```python
from build123d import *

# Parameters (mm, degrees)
SKETCH1_W           = 109.4
SKETCH1_H           = 109.4
SKETCH1_W_2         = 79.4
SKETCH1_H_2         = 79.4
SKETCH1_R           = 6
SKETCH1_R_2         = 1.5
BOSS_EXTRUDE1_DEPTH = 8
BOSS_EXTRUDE2_DEPTH = 109.4
FILLET1_R           = 30
SKETCH5_W           = 8
SKETCH5_H           = 149.4
BOSS_EXTRUDE3_DEPTH = 109.4
SKETCH3_W           = 8
SKETCH3_H           = 109.4
CUT_EXTRUDE4_DEPTH  = 135
SKETCH7_W           = 8
SKETCH7_H           = 40
CUT_EXTRUDE5_DEPTH  = 135
SKETCH4_R           = 2.5
CUT_EXTRUDE6_DEPTH  = 10


with BuildPart() as part:
    # Sketch1 → Boss-Extrude1 (new body)
    # profile 1 of 2: a face of its own
    with BuildSketch(Plane.XY):
        with Locations((-17.5, 17.5)):
            Rectangle(SKETCH1_W, SKETCH1_H)
        with Locations((-17.5, 17.5)):
            Rectangle(SKETCH1_W_2, SKETCH1_H_2, mode=Mode.SUBTRACT)
    # profile 2 of 2: a face of its own
    with BuildSketch(Plane.XY):
        with Locations((-17.5, 17.5)):
            Rectangle(SKETCH1_W_2, SKETCH1_H_2)
        with Locations((-35, 0)):
            Circle(SKETCH1_R, mode=Mode.SUBTRACT)
        Circle(SKETCH1_R, mode=Mode.SUBTRACT)
        with Locations((0, 35)):
            Circle(SKETCH1_R, mode=Mode.SUBTRACT)
        with Locations((-35, 35)):
            Circle(SKETCH1_R, mode=Mode.SUBTRACT)
        with Locations((-52.809903828, -17.809903828)):
            Circle(SKETCH1_R_2, mode=Mode.SUBTRACT)
        with Locations((-17.5, -17.5)):
            Circle(SKETCH1_R_2, mode=Mode.SUBTRACT)
        with Locations((17.5, -17.5)):
            Circle(SKETCH1_R_2, mode=Mode.SUBTRACT)
        with Locations((17.5, 17.5)):
            Circle(SKETCH1_R_2, mode=Mode.SUBTRACT)
        with Locations((-17.5, 17.5)):
            Circle(SKETCH1_R_2, mode=Mode.SUBTRACT)
        with Locations((-52.5, 17.5)):
            Circle(SKETCH1_R_2, mode=Mode.SUBTRACT)
        with Locations((17.5, 52.5)):
            Circle(SKETCH1_R_2, mode=Mode.SUBTRACT)
        with Locations((-17.5, 52.5)):
            Circle(SKETCH1_R_2, mode=Mode.SUBTRACT)
        with Locations((-52.5, 52.5)):
            Circle(SKETCH1_R_2, mode=Mode.SUBTRACT)
    extrude(amount=BOSS_EXTRUDE1_DEPTH)



with BuildPart() as body_2:
    # Sketch2 → Boss-Extrude2 (new body)
    with BuildSketch(Plane(origin=(37.2, 0, 0), x_dir=(0, 0, -1), z_dir=(1, 0, 0))):
        Polygon((-8, 72.2), (-33.651510749, 1.723053441), (-29.425328132, -7.340024429), (-32.127552961, -8.237713324), (-37.410281233, 3.091134014), (-12, 72.905307923), (-12, 112.2), (-8, 112.2), align=None)
    extrude(amount=-BOSS_EXTRUDE2_DEPTH)

    # Fillet1
    fillet1_edges = [body_2.edges().sort_by_distance(p)[0] for p in [
        (-17.5, 72.905307923, 12),
    ]]
    fillet(fillet1_edges, radius=FILLET1_R)


with BuildPart() as part_1:
    add(part.part)

    add(body_2.part)  # Boss-Extrude3 merges body 2
    # Sketch5 → Boss-Extrude3 (add)
    with BuildSketch(Plane(origin=(37.2, 0, 0), x_dir=(0, 0, -1), z_dir=(1, 0, 0))):
        with Locations((-4, 37.5)):
            Rectangle(SKETCH5_W, SKETCH5_H)
    extrude(amount=-BOSS_EXTRUDE3_DEPTH)

    # Sketch3 → Cut-Extrude4 (cut)
    with BuildSketch(Plane(origin=(37.2, 0, 0), x_dir=(0, 0, -1), z_dir=(1, 0, 0))):
        with Locations((-4, 17.5)):
            Rectangle(SKETCH3_W, SKETCH3_H)
    extrude(amount=-CUT_EXTRUDE4_DEPTH, mode=Mode.SUBTRACT)

    # Sketch7 → Cut-Extrude5 (cut)
    with BuildSketch(Plane(origin=(37.2, 0, 0), x_dir=(0, 0, -1), z_dir=(1, 0, 0))):
        with Locations((-4, 92.2)):
            Rectangle(SKETCH7_W, SKETCH7_H)
    extrude(amount=-CUT_EXTRUDE5_DEPTH, mode=Mode.SUBTRACT)

    # Sketch4 → Cut-Extrude6 (cut)
    with BuildSketch(Plane.XY.offset(12)):
        with Locations((-52.8, 94.2)):
            Circle(SKETCH4_R)
        with Locations((-32.8, 94.2)):
            Circle(SKETCH4_R)
        with Locations((-12.8, 94.2)):
            Circle(SKETCH4_R)
        with Locations((7.2, 94.2)):
            Circle(SKETCH4_R)
        with Locations((27.2, 94.2)):
            Circle(SKETCH4_R)
    extrude(amount=-CUT_EXTRUDE6_DEPTH, mode=Mode.SUBTRACT)


solid = part_1.part
```
The listing builds one solid part. Answer for the finished solid, in the listing's coordinates (mm). A direction names the side the tool comes from. Give positions to 0.01 mm unless a question says otherwise; leave off trailing zeros. Loops run counter-clockwise (first coordinate to the right, second up) from the corner with the lowest first, then second, coordinate; pieces in that order, holes last. Notation, with made-up numbers: M 28.25,81 L 62.25,81 A27 ccw 62.25,108 Z; hole C 33,42.25 d4. An arc over 180 degrees is marked long. One line per item, written item: value.
Q1. A cutting plane is placed at A-A on x = 26.5. Determine the outline of the cut face in (y, z).
Working result:
outline: M -8.24,32.13 L -7.34,29.43 L 1.72,33.65 L 72.2,8 L 91.8,8 L 91.8,12 L 78.2,12 A30 cw 67.93,13.81 L 3.09,37.41 Z; M 96.6,8 L 112.2,8 L 112.2,12 L 96.6,12 Z
Q2. A cutting plane is placed at D-D on z = 15.5. Determine the outline of the cut face in (x, y), then the cut area to 3 significant figures.
Working result:
outline: M -72.2,51.59 L 37.2,51.59 L 37.2,63.29 L -72.2,63.29 Z
area: 1,280 mm^2
Q3. A cutting plane is placed at C-C on x = 1.5. Determine the outline of the cut face in (y, z).
Working result:
outline: M -8.24,32.13 L -7.34,29.43 L 1.72,33.65 L 72.2,8 L 112.2,8 L 112.2,12 L 78.2,12 A30 cw 67.93,13.81 L 3.09,37.41 Z
Q4. Find the intervals of material crossed by line 1 (Z direction, x = 19, y = 92); line 2 (Z direction, x = -39, y = 34), in increasing order. Write a range as from..to.
Working result:
line 1: z = 8..12
line 2: z = 21.9..26.16
Q5. Flat-ended cylindrical pins translate along their axes: P1, Ø6.5, axis at x = -12.8, y = 94.2, coming from the +Z side; P2, Ø1, axis at x = 24.5, y = 63.5, coming from the +Z side; P3, Ø5, axis at x = -6, y = 19, coming from the -Z side; P4, Ø4.5, axis at x = 27.2, y = 94.2, coming from the -Z side. Find the tip coordinate at first contact, or state that the pin passes through.
Working result:
P1: stops at z = 12
P2: stops at z = 15.61
P3: stops at z = 26.45
P4: passes through
Q6. A cutting plane is placed at B-B on y = 94.2. Determine the outline of the cut face in (x, z), then the cut area to 3 significant figures.
Working result:
outline: M -72.2,8 L -55.3,8 L -55.3,12 L -72.2,12 Z; M -50.3,8 L -35.3,8 L -35.3,12 L -50.3,12 Z; M -30.3,8 L -15.3,8 L -15.3,12 L -30.3,12 Z; M -10.3,8 L 4.7,8 L 4.7,12 L -10.3,12 Z; M 9.7,8 L 24.7,8 L 24.7,12 L 9.7,12 Z; M 29.7,8 L 37.2,8 L 37.2,12 L 29.7,12 Z
area: 338 mm^2
Q7. Determine the mould class of faces 1 (the face through (-16.734, -2.653, 34.732)), 2 (the face through (-11.65, 91.98, 10.03)), 3 (the face through (-72.2, 52, 19)) for opening direction Y: +Y half, -Y half, draft (parallel to the pull), parting line (faces both ways), or undercut.
Working result:
face 1: -Y half
face 2: undercut
face 3: draft
Q8. For faces 4 (the face through (-17, 112.2, 10)), 5 (the face through (-16.734, -2.745, 31.568)), 6 (the face through (-17, 95, 12)), determine the directions among +Z, -Z, +X, -X, +Y, -Y from which every point of the face is accessible in a straight line to the end or side of a thin tool.
Working result:
face 4: +Z, -Z, +X, -X, +Y
face 5: -Z, +X, -X
face 6: +Z, +X, -X, +Y
